The listing builds one solid part. Answer for the finished solid, in the listing's coordinates (mm). Give positions to 0.01 mm unless a question says otherwise; leave off trailing zeros. Write each loop counter-clockwise with the first axis right and the second up, starting at its lowest first coordinate (ties: lowest second). Pieces come first, ordered by that corner, then holes. Notation, with made-up numbers: (86.25, -33) -> (98.25, -33) arc R18 cw to (98.25, -27) -> close; hole circle Ø5 at (4, 43.25). An arc over 180 degrees is marked (long way). Use CSV: the item, a comma, the result in double quotes. Start each with the question number.
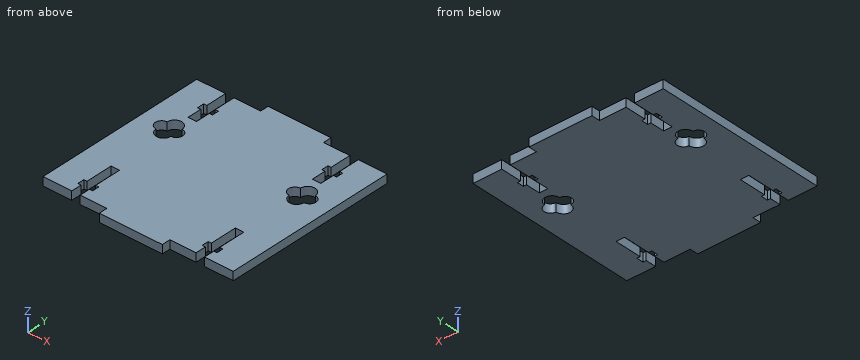
from build123d import *

# Parameters (mm, degrees)
SKETCH1_W           = 90
SKETCH1_H           = 82
BOSS_EXTRUDE1_DEPTH = 4
SKETCH4_W           = 29.8
SKETCH4_H           = 4
BOSS_EXTRUDE2_DEPTH = 4
CUT_EXTRUDE1_DEPTH  = 10
CUT_EXTRUDE2_DEPTH  = 10


with BuildPart() as part:
    # Sketch1 → Boss-Extrude1 (new body)
    with BuildSketch(Plane.XY):
        Rectangle(SKETCH1_W, SKETCH1_H)
    extrude(amount=BOSS_EXTRUDE1_DEPTH)

    # Sketch4 → Boss-Extrude2 (add)
    with BuildSketch(Plane.XY.offset(4)):
        with Locations((0.1, 43)):
            Rectangle(SKETCH4_W, SKETCH4_H)
    boss_extrude2 = extrude(amount=-BOSS_EXTRUDE2_DEPTH)

    # Mirror1: Boss-Extrude2 across plane
    add(boss_extrude2.mirror(Plane(origin=(0, 0, 0), x_dir=(0, 0, 1), z_dir=(0, -1, 0))))

    # Sketch5 → Cut-Extrude1 (cut)
    with BuildSketch(Plane.XY.offset(4)):
        Polygon((27.39999999, 41), (27.39999999, 31), (25.89999999, 31), (25.89999999, 27.8), (27.39999999, 27.8), (27.39999999, 21), (31.39999999, 21), (31.39999999, 27.8), (32.89999999, 27.8), (32.89999999, 31), (31.39999999, 31), (31.39999999, 41), align=None)
        Polygon((-27.39999999, 27.8), (-27.39999999, 21), (-31.39999999, 21), (-31.39999999, 27.8), (-32.89999999, 27.8), (-32.89999999, 31), (-31.39999999, 31), (-31.39999999, 41), (-27.39999999, 41), (-27.39999999, 31), (-25.89999999, 31), (-25.89999999, 27.8), align=None)
        Polygon((-27.4, -36), (-27.4, -41), (-31.4, -41), (-31.4, -36), (-32.9, -36), (-32.9, -32.8), (-31.4, -32.8), (-31.4, -20), (-27.4, -20), (-27.4, -32.8), (-25.9, -32.8), (-25.9, -36), align=None)
        Polygon((31.4, -41), (31.4, -36), (32.9, -36), (32.9, -32.8), (31.4, -32.8), (31.4, -20), (27.4, -20), (27.4, -32.8), (25.9, -32.8), (25.9, -36), (27.4, -36), (27.4, -41), align=None)
    extrude(amount=-CUT_EXTRUDE1_DEPTH, mode=Mode.SUBTRACT)

    # Sketch6 → Cut-Extrude2 (cut)
    with BuildSketch(Plane.XY.offset(4)):
        with BuildLine():
            ThreePointArc((27.96981837, 8.015850853), (25.015698228, 11), (27.96981837, 13.984149147))
            ThreePointArc((27.96981837, 13.984149147), (31.5, 17.463580565), (35.03018163, 13.984149147))
            ThreePointArc((35.03018163, 13.984149147), (37.984301772, 11), (35.03018163, 8.015850853))
            ThreePointArc((35.03018163, 8.015850853), (31.5, 4.536419435), (27.96981837, 8.015850853))
        make_face()
        with BuildLine():
            ThreePointArc((-27.96981837, 13.984149147), (-31.5, 17.463580565), (-35.03018163, 13.984149147))
            ThreePointArc((-35.03018163, 13.984149147), (-37.984301772, 11), (-35.03018163, 8.015850853))
            ThreePointArc((-35.03018163, 8.015850853), (-31.5, 4.536419435), (-27.96981837, 8.015850853))
            ThreePointArc((-27.96981837, 8.015850853), (-25.015698228, 11), (-27.96981837, 13.984149147))
        make_face()
    extrude(amount=-CUT_EXTRUDE2_DEPTH, mode=Mode.SUBTRACT)


solid = part.part
Q1. Straight lines are drawn through the part: L1, parallel to X at y = -29, z = 0.25; L2, parallel to X at y = 28, z = 1.15; L3, parallel to Y at x = 16.5, z = 1.6. For each, find the intervals that lie inside material, in ascending order.
Q2. Section A-A on y = 11 is taken. Give the vertices of the cut face in (x, z), then the cut area to 3 significant figures.
Q3. Section D-D on z = 2.95 is taken. State how many separate pieces and enclosed holes the cut face has, then the cut area to 3 significant figures.
Q4. Flat-ended cylindrical pins translate along their axes: pin 1 Ø0.8 at (x, z) = (-27, 2) entering from +Y; pin 2 Ø1.6 at (x, z) = (-32, 2) entering from -Y; pin 3 Ø8 at (x, y) = (-10, -5) entering from -Z; pin 4 Ø1.2 at (y, z) = (42.5, 1.5) entering from -X. Find the tip coordinate at first contact, or state that the pin passes through.
Q5. Section B-B on y = -38 is taken. Give the vertices of the cut face in (x, z).
Q6. Section C-C on x = -23.5 is taken. Give the vertices of the cut face in (y, z), then the cut area to 3 significant figures.
Output:
1,L1,"-45 to -31.4, -27.4 to 27.4, 31.4 to 45"
1,L2,"-45 to -32.9, -25.9 to 25.9, 32.9 to 45"
1,L3,"-41 to 41"
2,outline,"(-45, 0) -> (-37.98, 0) -> (-37.98, 4) -> (-45, 4) -> close; (-25.02, 0) -> (25.02, 0) -> (25.02, 4) -> (-25.02, 4) -> close; (37.98, 0) -> (45, 0) -> (45, 4) -> (37.98, 4) -> close"
2,area,"256 mm²"
3,separate pieces,"1"
3,enclosed holes,"2"
3,area,"7,040 mm²"
4,pin 1,"y = 41"
4,pin 2,"y = -41"
4,pin 3,"z = 0"
4,pin 4,"x = -14.8"
5,outline,"(-45, 0) -> (-31.4, 0) -> (-31.4, 4) -> (-45, 4) -> close; (-27.4, 0) -> (27.4, 0) -> (27.4, 4) -> (-27.4, 4) -> close; (31.4, 0) -> (45, 0) -> (45, 4) -> (31.4, 4) -> close"
6,outline,"(-41, 0) -> (41, 0) -> (41, 4) -> (-41, 4) -> close"
6,area,"328 mm²"
